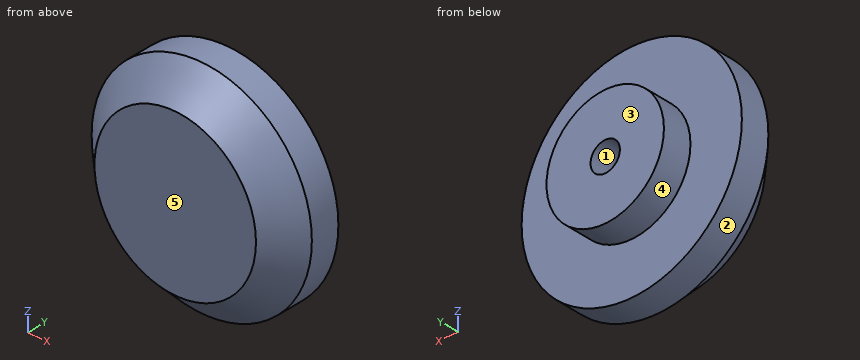
from build123d import *

# Parameters (mm, degrees)
F0_R     = 7.5
F1_DEPTH = 4
F2_R     = 4
F3_DEPTH = 2
F5_D     = 2
F5_DEPTH = 4
F5_TIP   = 0.600860619
F6_SIZE  = 2


with BuildPart() as f1:
    # F0 (on Front) → F1 (new body)
    with BuildSketch(Plane.XZ):
        Circle(F0_R)
    extrude(amount=F1_DEPTH)

    # F2 (on face) → F3 (join)
    with BuildSketch(Plane(origin=(0, 0, 0), x_dir=(-1, 0, 0), z_dir=(0, 1, 0))):
        Circle(F2_R)
    extrude(amount=F3_DEPTH)

    # F5
    with Locations(Plane(origin=(0, 2, 0), x_dir=(-1, 0, 0), z_dir=(0, 1, 0))):
        with Locations((0, 0)):
            Hole(F5_D / 2, depth=F5_DEPTH)
            with Locations((0, 0, -(F5_DEPTH + F5_TIP / 2))):  # 118° drill point
                Cone(0, F5_D / 2, F5_TIP, mode=Mode.SUBTRACT)

    # F6
    f6_edges = [f1.edges().sort_by_distance(p)[0] for p in [
        (-7.5, -4, 0),
    ]]
    chamfer(f6_edges, length=F6_SIZE)


solid = f1.part
Here's how the part is built. I have some questions about the finished solid (model axes, mm). Face numbers are marked on the shaded views. A direction names the side the tool comes from. Give positions to 0.01 mm unless a question says otherwise; leave off trailing zeros. Loops run counter-clockwise (first coordinate to the right, second up) from the corner with the lowest first, then second, coordinate; pieces in that order, holes last. Notation, with made-up numbers: (-1, 50.25) -> (41, 50.25) arc R18 ccw to (41, 64.25) -> close; hole circle Ø8 at (16.5, -3). An arc over 180 degrees is marked (long way). One line per item, written item: value.
Q1. We'd pull the mould along X, two halves only. Please class the marked faces 1, 2 and 3: pulls with the +X half, pulls with the -X half, needs draft (parallel to the pull), parting line crosses it, or undercut.
Answers follow:
face 1: undercut
face 2: parting line crosses it
face 3: needs draft
Q2. If I drill on line 1 along Z through (x, y) = (0, 0.9); line 2 along Y through (x, z) = (-2.25, -3.5); line 3 along Y through (x, z) = (-1.25, 5.75), over which ranges is the centre line in solid material (lowest first)?
Answers follow:
line 1: -4 to -1, 1 to 4
line 2: -4 to 0
line 3: -3.62 to 0
Q3. I'm going to push flat-ended pins straight in: pin 1 Ø2 at (y, z) = (-3, -3.5) entering from -X; pin 2 Ø1.5 at (x, y) = (4, 1) entering from +Z. Where does each tip first touch, or does it pass through?
Answers follow:
pin 1: x = -6.74
pin 2: z = 2.33
Q4. Suppose I cut it at A-A on y = -1.3. Please give me the cut outline in (x, z), then the cut area to 3 significant figures.
Answers follow:
outline: circle Ø15 at (0, 0); hole circle Ø2 at (0, 0)
area: 174 mm^2
Q5. On a 3-axis mill with a long thin cutter (end or side, diameter ignored), from which of +Z, -Z, +X, -X, +Y, -Y can I reach the whole of each face in a straight line? I mean the marked faces 4 and 5. Say none if no direction works.
Answers follow:
face 4: +Y
face 5: +Z, -Z, +X, -X, -Y
